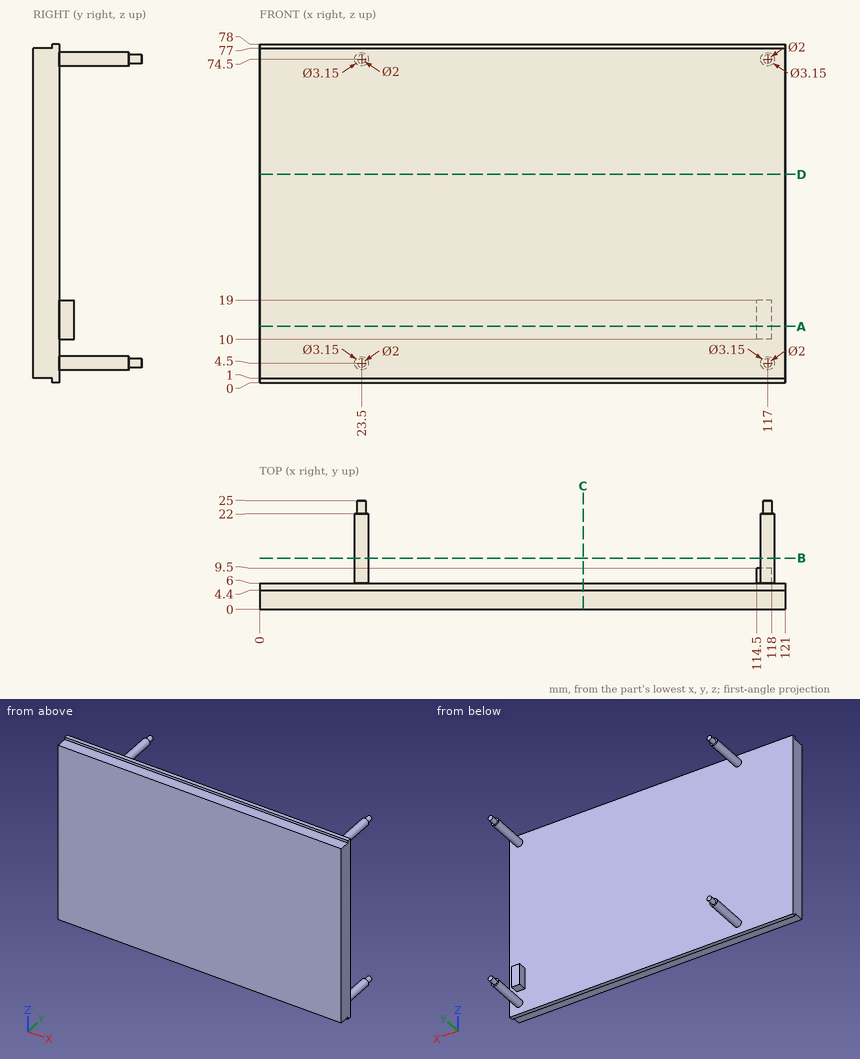
Source: three-view drawing plus pictorial views. Frame: mm from the lowest corner of the part. Coordinates: 2 decimals unless noted, no trailing zeros. Loops run counter-clockwise (first coordinate to the right, second up) from the corner with the lowest first, then second, coordinate; pieces in that order, holes last. Notation, with made-up numbers: (-11, 20) - (42, 20) arc R23 ccw to (42, 37) - close; hole circle Ø6 at (-11, -40). An arc over 180 degrees is marked (long way). One line per item, written item: value. Start each with the question number.
1. Section D-D (z = 48). Return the cut outline in (x, y), and give its area (3 significant figures).
2. Contact query for flat-ended pins moving along their axis: P1, Ø2, axis at x = 74.5, y = 2.5, coming from the -Z side; P2, Ø0.5, axis at x = 46, z = 77.5, coming from the -Y side; P3, Ø3, axis at x = 117, z = 12.5, coming from the +Y side. Output: stop coordinate, or through.
3. Section B-B (y = 11.75). Return the cut outline in (x, z) (3 decimals), and give its area (3 significant figures).
4. Ray query, L1, parallel to Y at x = 62.5, z = 72; L2, parallel to X at y = 23, z = 5; L3, parallel to Z at x = 10, y = 3. Return the intervals inside material, ascending.
5. Section A-A (z = 13). Return the cut outline in (x, y).
6. Section C-C (x = 74.5). Return the cut outline in (y, z), and give its area (3 significant figures).
Verdict:
1. outline: (0, 0) - (121, 0) - (121, 6) - (0, 6) - close
1. area: 726 mm2
2. P1: stops at z = 1
2. P2: stops at y = 4.4
2. P3: stops at y = 9.5
3. outline: circle Ø3.15 at (23.5, 4.5); circle Ø3.15 at (23.5, 74.5); circle Ø3.15 at (117, 4.5); circle Ø3.15 at (117, 74.5)
3. area: 31.2 mm2
4. L1: y = 0 to 6
4. L2: x = 22.63 to 24.37, 116.13 to 117.87
4. L3: z = 1 to 77
5. outline: (0, 0) - (121, 0) - (121, 6) - (118, 6) - (118, 9.5) - (114.5, 9.5) - (114.5, 6) - (0, 6) - close
6. outline: (0, 1) - (4.4, 1) - (4.4, 0) - (6, 0) - (6, 78) - (4.4, 78) - (4.4, 77) - (0, 77) - close
6. area: 459 mm2
